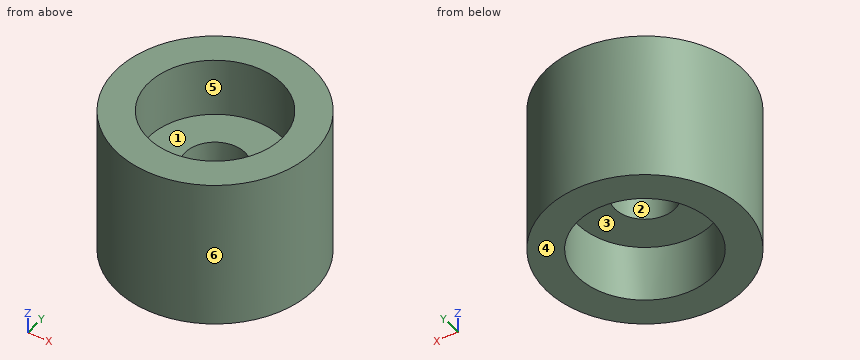
from build123d import *

# Parameters (mm, degrees)
F0_R     = 16.5
F0_R_2   = 5
F1_DEPTH = 25
F2_R     = 11.15
F3_DEPTH = 9.75
F4_R     = 11.225
F5_DEPTH = 9.5


with BuildPart() as f1:
    # F0 (on Top) → F1 (new body)
    with BuildSketch(Plane.XY):
        Circle(F0_R)
        Circle(F0_R_2, mode=Mode.SUBTRACT)
    extrude(amount=F1_DEPTH)

    # F2 (on face) → F3 (cut)
    with BuildSketch(Plane.XY.offset(25)):
        Circle(F2_R)
    extrude(amount=-F3_DEPTH, mode=Mode.SUBTRACT)

    # F4 (on Top) → F5 (cut)
    with BuildSketch(Plane.XY):
        Circle(F4_R)
    extrude(amount=F5_DEPTH, mode=Mode.SUBTRACT)


solid = f1.part
Read the model definition and answer for the solid it produces. Units are mm, in the model's axes. Face numbers are marked on the shaded views. A direction names the side the tool comes from. Round coordinates to 2 decimals unless told otherwise and drop trailing zeros. Write each loop counter-clockwise with the first axis right and the second up, starting at its lowest first coordinate (ties: lowest second). Pieces come first, ordered by that corner, then holes.
1. Which of the six approach directions +Z, -Z, +X, -X, +Y, -Y give full straight-line access (tool end or side, diameter ignored) to the marked faces 1, 2 and 3?
2. The part is cut by section D-D, the plane y = -9.5. Determine the outline of the cut face in (x, z).
3. The part is cut by section B-B, the plane y = -1. Determine the outline of the cut face in (x, z).
4. Straight lines are drawn through the part: L1, parallel to Y at x = 0, z = 6.5 (3 decimals); L2, parallel to Y at x = 0, z = 18.75; L3, parallel to X at y = -9.5, z = 5.25. For each, find the intervals that lie inside material, in ascending order.
5. Given pin 1 Ø1 at (x, z) = (-13, 8.5) entering from -Y; pin 2 Ø6.5 at (x, y) = (0.5, 2) entering from +Z; pin 3 Ø8 at (x, z) = (10, 5) entering from -Y, each flat-ended and moving along its own axis, determine where each tip first touches the part or whether it passes through.
6. The part is cut by section C-C, the plane z = 3.75. Determine the outline of the cut face in (x, y) (3 decimals).
7. Determine the mould class of the marked faces 4, 5 and 6 for opening direction X: pulls with the +X half, pulls with the -X half, needs draft (parallel to the pull), parting line crosses it, or undercut.
8. The part is cut by section A-A, the plane x = 0. Determine the outline of the cut face in (y, z) (3 decimals), then the cut area to 3 significant figures.
Values:
1. face 1: +Z
1. face 2: +Z, -Z
1. face 3: -Z
2. outline: (-13.49, 0) - (-5.98, 0) - (-5.98, 9.5) - (5.98, 9.5) - (5.98, 0) - (13.49, 0) - (13.49, 25) - (5.84, 25) - (5.84, 15.25) - (-5.84, 15.25) - (-5.84, 25) - (-13.49, 25) - close
3. outline: (-16.47, 0) - (-11.18, 0) - (-11.18, 9.5) - (-4.9, 9.5) - (-4.9, 15.25) - (-11.11, 15.25) - (-11.11, 25) - (-16.47, 25) - close; (4.9, 9.5) - (11.18, 9.5) - (11.18, 0) - (16.47, 0) - (16.47, 25) - (11.11, 25) - (11.11, 15.25) - (4.9, 15.25) - close
4. L1: y = -16.5 to -11.225, 11.225 to 16.5
4. L2: y = -16.5 to -11.15, 11.15 to 16.5
4. L3: x = -13.49 to -5.98, 5.98 to 13.49
5. pin 1: stops at y = -10.77
5. pin 2: stops at z = 15.25
5. pin 3: stops at y = -15.37
6. outline: circle Ø33 at (0, 0); hole circle Ø22.45 at (0, 0)
7. face 4: needs draft
7. face 5: undercut
7. face 6: parting line crosses it
8. outline: (-16.5, 0) - (-11.225, 0) - (-11.225, 9.5) - (-5, 9.5) - (-5, 15.25) - (-11.15, 15.25) - (-11.15, 25) - (-16.5, 25) - close; (5, 9.5) - (11.225, 9.5) - (11.225, 0) - (16.5, 0) - (16.5, 25) - (11.15, 25) - (11.15, 15.25) - (5, 15.25) - close
8. area: 337 mm2
